Geometry check sheet. Reference: drawing and pictorial views, mm from the part's lowest x, y, z. A direction names the side the tool comes from. Round coordinates to 2 decimals unless told otherwise and drop trailing zeros. Write each loop counter-clockwise with the first axis right and the second up, starting at its lowest first coordinate (ties: lowest second). Pieces come first, ordered by that corner, then holes. Notation, with made-up numbers: (-39, -40) -> (-12, -40) arc R35 ccw to (-12, -6) -> close; hole circle Ø7 at (-32.5, 9.5). An arc over 180 degrees is marked (long way). Answer as a JSON object with one key per item and string values. Group by question number.
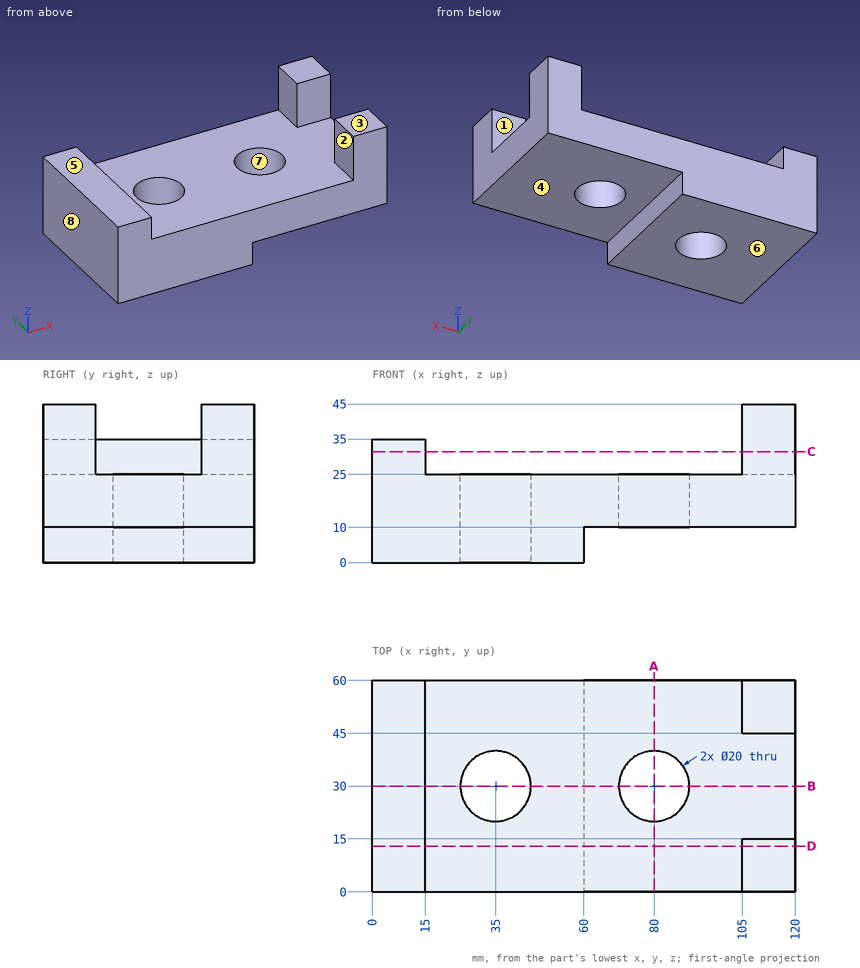
(1) Access from +Z, -Z, +X, -X, +Y, -Y to the whole of each face (thin tool, end or side, straight path). Record for the marked faces 1, 2, 3, 4 and 5.
(2) Section check B-B on y = 30. Record the cut outline in (x, z), then the cut area to 3 significant figures.
(3) Release check for a two-part mould opening along X. For the marked faces 6, 7 and 8 record: pulls with the +X half, pulls with the -X half, needs draft (parallel to the pull), parting line crosses it, or undercut.
(4) Scan lines: line 1 along Y through (x, z) = (80, 14.25); line 2 along X through (y, z) = (24.5, 13.5); line 3 along X through (y, z) = (36, 15.5). Record each from-to range of solid material in increasing order.
(5) Go/stop test with flat-tipped pins: pin 1 Ø16.5 at (x, y) = (6.5, 26) entering from +Z; pin 2 Ø3 at (y, z) = (21.5, 3) entering from +X; pin 3 Ø3 at (y, z) = (36, 31.5) entering from +X; pin 4 Ø12 at (x, y) = (80, 30) entering from -Z. Record where each tip stops, or that it passes through.
(6) Section check A-A on x = 80. Record the cut outline in (y, z).
(7) Section check C-C on z = 31.5. Record the cut outline in (x, y).
(8) Section check D-D on y = 13. Record the cut outline in (x, z), then the cut area to 3 significant figures.
Data:
{
 "1": {"face 1": "+Z, +X", "face 2": "+Z, +Y, -Y", "face 3": "+Z, +X, -X, +Y, -Y", "face 4": "-Z, +X, +Y, -Y", "face 5": "+Z, -X, +Y, -Y"},
 "2": {"outline": "(0, 0) -> (25, 0) -> (25, 25) -> (15, 25) -> (15, 35) -> (0, 35) -> close; (45, 0) -> (60, 0) -> (60, 10) -> (70, 10) -> (70, 25) -> (45, 25) -> close; (90, 10) -> (120, 10) -> (120, 25) -> (90, 25) -> close", "area": "1,750 mm²"},
 "3": {"face 6": "needs draft", "face 7": "undercut", "face 8": "pulls with the -X half"},
 "4": {"line 1": "y = 0 to 20, 40 to 60", "line 2": "x = 0 to 26.65, 43.35 to 71.65, 88.35 to 120", "line 3": "x = 0 to 27, 43 to 72, 88 to 120"},
 "5": {"pin 1": "stops at z = 35", "pin 2": "stops at x = 60", "pin 3": "stops at x = 15", "pin 4": "passes through"},
 "6": {"outline": "(0, 10) -> (20, 10) -> (20, 25) -> (0, 25) -> close; (40, 10) -> (60, 10) -> (60, 25) -> (40, 25) -> close"},
 "7": {"outline": "(0, 0) -> (15, 0) -> (15, 60) -> (0, 60) -> close; (105, 0) -> (120, 0) -> (120, 15) -> (105, 15) -> close; (105, 45) -> (120, 45) -> (120, 60) -> (105, 60) -> close"},
 "8": {"outline": "(0, 0) -> (60, 0) -> (60, 10) -> (120, 10) -> (120, 45) -> (105, 45) -> (105, 25) -> (15, 25) -> (15, 35) -> (0, 35) -> close", "area": "2,850 mm²"}
}
